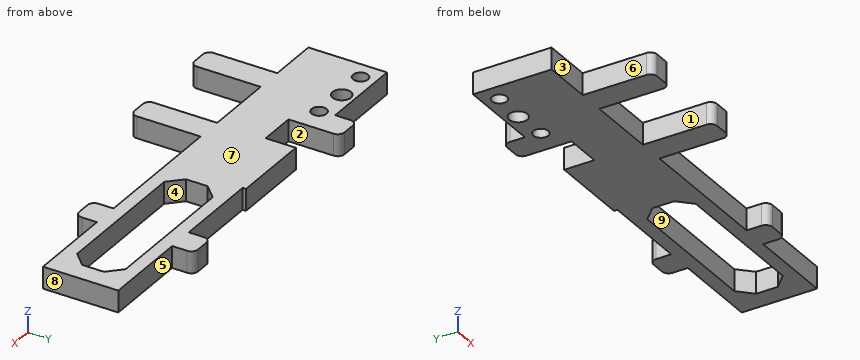
Autodesk Inventor part; units mm, degrees
ref_plane "YZ Plane" through (0, 0, 0) normal (1, 0, 0) x (0, 1, 0)
ref_plane "XZ Plane" through (0, 0, 0) normal (0, 1, 0) x (-1, 0, 0)
ref_plane "XY Plane" through (0, 0, 0) normal (0, 0, 1) x (1, 0, 0)
sketch "Sketch1" plane through (0, 0, 0) normal (0, 0, 1) x (1, 0, 0)
  line L0 (0, 0) -> (128, 0)
  line L1 (128, 0) -> (128, 22.5)
  line L2 (0, 23.5) -> (0, 0)
  line L3 (68, 23.5) -> (68, 22.5)
  line L4 (68, 22.5) -> (128, 22.5)
  line L5 (33, 23.5) -> (33, 14.5)
  line L6 (33, 14.5) -> (44, 14.5)
  line L7 (44, 14.5) -> (44, 23.5)
  line L8 (68, 23.5) -> (44, 23.5)
  line L9 (33, 23.5) -> (0, 23.5)
  line L10 (72, 14.5) -> (72, 8)
  line L11 (72, 8) -> (76, 4)
  line L12 (76, 4) -> (118, 4)
  line L13 (118, 4) -> (122, 8)
  line L14 (122, 8) -> (122, 14.5)
  line L15 (122, 14.5) -> (118, 18.5)
  line L16 (118, 18.5) -> (76, 18.5)
  line L17 (76, 18.5) -> (72, 14.5)
  line L18 (68, 22.5) -> (68, 0) construction
  circle A0 centre (5.5, 19) radius 2.25
  circle A1 centre (25.5, 19) radius 2.25
  circle A2 centre (15.5, 19.599) radius 2.75
  circle A3 centre (38.5, 19.599) radius 7.5 construction
  circle A4 centre (38.5, 19.599) radius 4 construction
  point P0 (33, 19)
  dimension "d0" = 128
  dimension "d1" = 23.5
  dimension "d2" = 22.5
  dimension "d3" = 60
  dimension "d4" = 11
  dimension "d5" = 9
  dimension "d6" = 33
  dimension "d7" = 45
  dimension "d8" = 4
  dimension "d9" = 4
  dimension "d10" = 6
  dimension "d11" = 4
  dimension "d12" = 4
  dimension "d13" = 4.5
  dimension "d14" = 4.5
  dimension "d15" = 5.5
  dimension "d16" = 20
  dimension "d17" = 5.5
  dimension "d18" = 8
  dimension "d19" = 15
  dimension "d20" = 10
extrude "Extrusion1" add sketch "Sketch1" along normal blind 6.5
sketch "Sketch2" plane through (0, 0, 6.5) normal (0, 0, 1) x (1, 0, 0)
  line L0 (0, 0) -> (128, 0)
  line L1 (128, 0) -> (128, 22.5)
  line L2 (128, 22.5) -> (68, 22.5)
  line L3 (33, 23.5) -> (0, 23.5)
  line L4 (0, 23.5) -> (0, 0)
  line L5 (25, 23.5) -> (33, 23.5)
  line L6 (33, 23.5) -> (33, 28)
  line L7 (31, 30) -> (27, 30)
  line L8 (25, 28) -> (25, 23.5)
  line L9 (94, 22.5) -> (102, 22.5)
  line L10 (102, 22.5) -> (102, 27)
  line L11 (100, 29) -> (96, 29)
  line L12 (94, 27) -> (94, 22.5)
  line L13 (15, 0) -> (23, 0)
  line L14 (23, 0) -> (23, -19)
  line L15 (21, -21) -> (17, -21)
  line L16 (15, -19) -> (15, 0)
  line L17 (44, 0) -> (52, 0)
  line L18 (52, 0) -> (52, -19)
  line L19 (50, -21) -> (46, -21)
  line L20 (44, -19) -> (44, 0)
  line L21 (94, 0) -> (102, 0)
  line L22 (102, 0) -> (102, -4.5)
  line L23 (100, -6.5) -> (96, -6.5)
  line L24 (94, -4.5) -> (94, 0)
  arc A0 (27, 30) -> (25, 28) centre (27, 28) ccw
  arc A1 (33, 28) -> (31, 30) centre (31, 28) ccw
  arc A2 (96, 29) -> (94, 27) centre (96, 27) ccw
  arc A3 (102, 27) -> (100, 29) centre (100, 27) ccw
  arc A4 (15, -19) -> (17, -21) centre (17, -19) ccw
  arc A5 (21, -21) -> (23, -19) centre (21, -19) ccw
  arc A6 (44, -19) -> (46, -21) centre (46, -19) ccw
  arc A7 (50, -21) -> (52, -19) centre (50, -19) ccw
  arc A8 (94, -4.5) -> (96, -6.5) centre (96, -4.5) ccw
  arc A9 (100, -6.5) -> (102, -4.5) centre (100, -4.5) ccw
  line L25 (33, 14.5) -> (33, 23.5)
  dimension "d23" = 2
  dimension "d24" = 8
  dimension "d25" = 8
  dimension "d26" = 8
  dimension "d27" = 8
  dimension "d28" = 8
  dimension "d29" = 21
  dimension "d30" = 6.5
  dimension "d31" = 6.5
  dimension "d33" = 26
  dimension "d34" = 15
  dimension "d35" = 21
  dimension "d38" = 6.5
extrude "Extrusion2" add sketch "Sketch2" against normal blind 6.5
properties part number "x_iddler_upper_nut_stop"
Source: CAD feature listing. Evaluate the final solid. Frame: model axes, mm. Face numbers are marked on the shaded views. A direction names the side the tool comes from. Coordinates: 2 decimals unless noted, no trailing zeros. Loops run counter-clockwise (first coordinate to the right, second up) from the corner with the lowest first, then second, coordinate; pieces in that order, holes last. Notation, with made-up numbers: (-28, 20) - (8, 20) arc R22 ccw to (8, 59) - close; hole circle Ø2 at (7.5, 45). An arc over 180 degrees is marked (long way). One line per question, with ' | ' between items.
1) First-contact query: P1, Ø2, axis at x = 35, z = 0.5, coming from the -Y side; P2, Ø2, axis at y = -5, z = 2, coming from the +X side; P3, Ø3, axis at x = 75.5, z = 2.5, coming from the +Y side. Flat tips, straight axial feed; report the tip coordinate or a pass-through.
Report:
P1: stops at y = 0 | P2: stops at x = 102 | P3: stops at y = 22.5
2) Line query: line 1 along X through (y, z) = (-4, 5); line 2 along X through (y, z) = (10.5, 5.75); line 3 along X through (y, z) = (-10, 6.25). Output: solid intervals per line, ascending.
Report:
line 1: x = 15 to 23, 44 to 52, 94 to 102 | line 2: x = 0 to 72, 122 to 128 | line 3: x = 15 to 23, 44 to 52
3) Section A-A, the plane x = 5.5. Return loops of the section in (y, z), then the cut area to 4 significant figures.
Report:
outline: (0, 0) - (16.75, 0) - (16.75, 6.5) - (0, 6.5) - close; (21.25, 0) - (23.5, 0) - (23.5, 6.5) - (21.25, 6.5) - close | area: 123.5 mm²
4) Section B-B, the plane x = 54. Return loops of the section in (y, z).
Report:
outline: (0, 0) - (23.5, 0) - (23.5, 6.5) - (0, 6.5) - close
5) Pull-direction query (X, two-part tool) for the marked faces 6, 7, 8 and 9; classes: released by +X, released by -X, zero draft, split by the parting line, or undercut.
Report:
face 6: released by -X | face 7: zero draft | face 8: released by +X | face 9: undercut
6) Set-up query: the marked faces 1, 2, 3, 4 and 5. Return all of +Z, -Z, +X, -X, +Y, -Y with unobstructed straight access to the full face (end or side cutting, diameter ignored); none if empty.
Report:
face 1: +Z, -Z, -Y | face 2: +Z, -Z, +Y | face 3: +Z, -Z, -X, -Y | face 4: +Z, -Z | face 5: +Z, -Z, +X, +Y
7) Section C-C, the plane z = 4.75. Give the number of separate pieces and of enclosed holes in the cut face, then the cut area to 3 significant figures.
Report:
separate pieces: 1 | enclosed holes: 4 | area: 2,580 mm²
